Input: part model. Units: mm. Frame: model coordinates. Face numbers are marked on the shaded views. A direction names the side the tool comes from. Give positions to 0.01 mm unless a question says otherwise; leave off trailing zeros. Loops run counter-clockwise (first coordinate to the right, second up) from the corner with the lowest first, then second, coordinate; pieces in that order, holes last. Notation, with made-up numbers: (64, 42.5) - (111, 42.5) arc R18 cw to (111, 55.5) - close; hole circle Ø7 at (15, 72.25). An arc over 180 degrees is marked (long way). Answer as a JSON object with one key per item and string values.
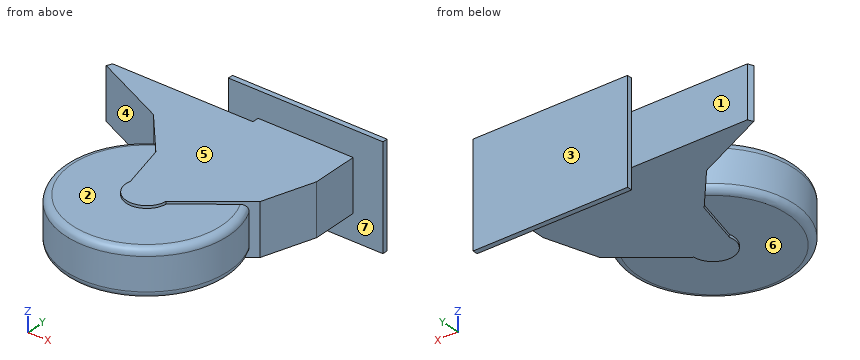
from build123d import *

# Parameters (mm, degrees)
SKETCH1_R                = 47.5
BOSS_EXTRUDE1_DEPTH      = 13.5
BOSS_EXTRUDE1_DEPTH_BACK = 13.5
FILLET1_R                = 4
BOSS_EXTRUDE2_DEPTH      = 15
BOSS_EXTRUDE2_DEPTH_BACK = 15
SKETCH5_W                = 90
SKETCH5_H                = 60
BOSS_EXTRUDE3_DEPTH      = 3


with BuildPart() as part:
    # Sketch1 → Boss-Extrude1 (new body, two sides)
    with BuildSketch(Plane.XY) as boss_extrude1_sk:
        Circle(SKETCH1_R)
    extrude(amount=BOSS_EXTRUDE1_DEPTH)
    extrude(boss_extrude1_sk.sketch, amount=-BOSS_EXTRUDE1_DEPTH_BACK)

    # Fillet1
    fillet1_edges = [part.edges().sort_by_distance(p)[0] for p in [
        (-47.5, 0, 13.5),
        (-47.5, 0, -13.5),
    ]]
    fillet(fillet1_edges, radius=FILLET1_R)

    # Sketch2 → Boss-Extrude2 (add, two sides)
    with BuildSketch(Plane.XY) as boss_extrude2_sk:
        with BuildLine():
            Line((-11.696785431, 2.681397647), (-18.496519497, 30.047194196))
            Line((-18.496519497, 30.047194196), (-39.614315725, 55.004751509))
            Line((-39.614315725, 55.004751509), (-83.032226589, 75.23))
            Line((-83.032226589, 75.23), (-81.634744669, 78.23))
            Line((-81.634744669, 78.23), (0, 78.23))
            Line((0, 78.23), (0, 82.04))
            Line((0, 82.04), (55.339662837, 82.04))
            Line((55.339662837, 82.04), (55.339662837, 55.004751509))
            Line((55.339662837, 55.004751509), (45.787278668, 25.414095095))
            Line((45.787278668, 25.414095095), (11.963303828, -0.940236292))
            ThreePointArc((11.963303828, -0.940236292), (-1.815713665, -11.862034676), (-11.696785431, 2.681397647))
        make_face()
    extrude(amount=BOSS_EXTRUDE2_DEPTH)
    extrude(boss_extrude2_sk.sketch, amount=-BOSS_EXTRUDE2_DEPTH_BACK)

    # Sketch5 → Boss-Extrude3 (add)
    with BuildSketch(Plane(origin=(0, 82.04, 0), x_dir=(1, 0, 0), z_dir=(0, 1, 0))):
        with Locations((27.669831419, 0)):
            Rectangle(SKETCH5_W, SKETCH5_H)
    extrude(amount=BOSS_EXTRUDE3_DEPTH)


solid = part.part
Item 1: Cut plane A-A (x = 57.5). Return loops of the section in (y, z).
Geometry check:
{"outline": "(82.04, -30) - (85.04, -30) - (85.04, 30) - (82.04, 30) - close"}
Item 2: Contact query for flat-ended pins moving along their axis: P1, Ø6, axis at x = -55.5, z = 2, coming from the +Y side; P2, Ø5, axis at x = 17.5, y = 36, coming from the +Z side; P3, Ø2.5, axis at y = 83.5, z = 0, coming from the -X side. Output: stop coordinate, or through.
Geometry check:
{"P1": "stops at y = 78.23", "P2": "stops at z = 15", "P3": "stops at x = -17.33"}
Item 3: Access query for the marked faces 4, 5, 6 and 7. Directions: +Z, -Z, +X, -X, +Y, -Y. A direction counts if a zero-diameter tool reaches every point of the face in a straight line with its end or side. Return the directions, or none.
Geometry check:
{"face 4": "+Z, -Z, -X", "face 5": "+Z, +X, -X, -Y", "face 6": "-Z, -Y", "face 7": "none"}
Item 4: Mould query, pull axis Y, two halves, no side actions, for the marked faces 1, 2 and 3. Classes: released by +Y, released by -Y, zero draft, split by the parting line, or undercut.
Geometry check:
{"face 1": "undercut", "face 2": "zero draft", "face 3": "released by +Y"}
Item 5: Cut plane C-C (z = 6). Return loops of the section in (x, y), then the cut area to 3 significant figures.
Geometry check:
{"outline": "(-83.03, 75.23) - (-39.61, 55) - (-26.45, 39.45) arc R47.5 ccw (long way) to (41.9, 22.38) - (45.79, 25.41) - (55.34, 55) - (55.34, 82.04) - (72.67, 82.04) - (72.67, 85.04) - (-17.33, 85.04) - (-17.33, 82.04) - (0, 82.04) - (0, 78.23) - (-81.63, 78.23) - close", "area": "11,600 mm2"}
Item 6: Cut plane B-B (z = 25.5). Return loops of the section in (x, y).
Geometry check:
{"outline": "(-17.33, 82.04) - (72.67, 82.04) - (72.67, 85.04) - (-17.33, 85.04) - close"}
Item 7: Material intervals for line 1 (Z direction, x = 30, y = 69.5); line 2 (X direction, y = -0.5, z = 1); line 3 (Y direction, x = 27, z = 16), sorted ascending. Write a range as [from, to].
Geometry check:
{"line 1": "z = [-15, 15]", "line 2": "x = [-47.5, 47.5]", "line 3": "y = [82.04, 85.04]"}
